Can you work these out from the model? Positions are in its coordinate system, mm. Give positions to 0.01 mm unless a question says otherwise; leave off trailing zeros. Loops run counter-clockwise (first coordinate to the right, second up) from the corner with the lowest first, then second, coordinate; pieces in that order, holes last. Notation, with made-up numbers: (85.25, -18.75) - (118.25, -18.75) arc R17 ccw to (118.25, 2.25) - close; hole circle Ø5 at (54.5, 33.25). An arc over 180 degrees is marked (long way). Answer as a JSON object with one key per item and string values. Group by question number.
Item 1: Suppose I cut it at A-A on x = -38.1. Write out the boundary of the cut face in (y, z), and give its area (3 significant figures).
Item 2: Thinking about a two-plate mould opening in X: for faces 1 (the cylindrical face through (0.58, -6.26, 60.23)), 2 (the flat face through (-12, 0, -7)), 3 (the cylindrical face through (2.753, -6.439, 56.765)), which applies, pulls with the +X half, pulls with the -X half, needs draft (parallel to the pull), parting line crosses it, or undercut?
Item 3: Suppose I cut it at D-D on z = -14. Write out the boundary of the cut face in (x, y).
Item 4: Suppose I cut it at B-B on x = 0. Write out the boundary of the cut face in (y, z), and give its area (3 significant figures).
Item 5: Will these pins go through, and if not, where does the flat tip stop? pin 1 (15 mm diameter, centred on x = 38.1, z = -21.62, fed in from -Y); pin 2 (4 mm diameter, centred on x = -28, y = -4, fed in from -Z); pin 3 (1 mm diameter, centred on y = -5, z = 4, fed in from -X); pin 4 (6 mm diameter, centred on x = -39.5, y = -11, fed in from +Z).
Item 6: Suppose I cut it at C-C on z = 11. Write out the boundary of the cut face in (x, y), and give its area (3 significant figures).
Item 7: Please list where these lines run through material, in increasing order: L1, parallel to Z at x = 0, y = -5.75; L2, parallel to Z at x = -38.1, y = -8.5; L3, parallel to X at y = -11, z = -22.
from build123d import *

# Parameters (mm, degrees)
F0_R     = 15.7260613119
F1_DEPTH = 12.7
F2_D     = 25.4


with BuildPart() as f1:
    # F0 (on Front) → F1 (new body)
    with BuildSketch(Plane.XZ):
        with BuildLine():
            ThreePointArc((-22.225, -21.624488881), (-24.3518467149, -13.686988881), (-30.1625, -7.8763355959))
            ThreePointArc((-30.1625, -7.8763355959), (-51.8481532851, -29.561988881), (-22.225, -21.624488881))
        make_face()
        with BuildLine():
            ThreePointArc((7.9375, 30.6184936023), (0, 28.4916468874), (-7.9375, 30.6184936023))
            ThreePointArc((-7.9375, 30.6184936023), (-15.8714708467, 9.5359543409), (-30.1625, -7.8763355959))
            ThreePointArc((-30.1625, -7.8763355959), (-24.3518467149, -13.686988881), (-22.225, -21.624488881))
            ThreePointArc((-22.225, -21.624488881), (0, -17.2054544996), (22.225, -21.624488881))
            ThreePointArc((22.225, -21.624488881), (24.3518467149, -13.686988881), (30.1625, -7.8763355959))
            ThreePointArc((30.1625, -7.8763355959), (15.3716015359, 9.2473546597), (7.9375, 30.6184936023))
        make_face()
        with Locations((0, 0.3947862569)):
            Circle(F0_R, mode=Mode.SUBTRACT)
        with BuildLine():
            ThreePointArc((53.975, -21.624488881), (46.0375, -7.8763355959), (30.1625, -7.8763355959))
            ThreePointArc((30.1625, -7.8763355959), (24.3518467149, -13.686988881), (22.225, -21.624488881))
            ThreePointArc((22.225, -21.624488881), (38.1, -37.499488881), (53.975, -21.624488881))
        make_face()
        with Locations((0, 0.3947862569)):
            Circle(F0_R)
        with BuildLine():
            ThreePointArc((7.9375, 30.6184936023), (13.7481532851, 36.4291468874), (15.875, 44.3666468874))
            ThreePointArc((15.875, 44.3666468874), (-7.9375, 58.1148001724), (-7.9375, 30.6184936023))
            ThreePointArc((-7.9375, 30.6184936023), (0, 28.4916468874), (7.9375, 30.6184936023))
        make_face()
    extrude(amount=F1_DEPTH)

    # F2 (through all)
    with Locations(Plane(origin=(0, 0, 0), x_dir=(1, 0, 0), z_dir=(0, 1, 0))):
        with Locations((-38.1, 21.624488881), (38.1, 21.624488881), (0, -44.3666468874), (0, -0.3947862569)):
            Hole(F2_D / 2)


solid = f1.part
Worked out:
{
 "1": {"outline": "(-12.7, -37.5) - (0, -37.5) - (0, -34.32) - (-12.7, -34.32) - close; (-12.7, -8.92) - (0, -8.92) - (0, -5.75) - (-12.7, -5.75) - close", "area": "80.6 mm2"},
 "2": {"face 1": "parting line crosses it", "face 2": "needs draft", "face 3": "undercut"},
 "3": {"outline": "(-52.02, -12.7) - (-48.26, -12.7) - (-48.26, 0) - (-52.02, 0) - close; (-27.94, -12.7) - (27.94, -12.7) - (27.94, 0) - (-27.94, 0) - close; (48.26, -12.7) - (52.02, -12.7) - (52.02, 0) - (48.26, 0) - close"},
 "4": {"outline": "(-12.7, -17.21) - (0, -17.21) - (0, -12.31) - (-12.7, -12.31) - close; (-12.7, 13.09) - (0, 13.09) - (0, 31.67) - (-12.7, 31.67) - close; (-12.7, 57.07) - (0, 57.07) - (0, 60.24) - (-12.7, 60.24) - close", "area": "338 mm2"},
 "5": {"pin 1": "passes through", "pin 2": "stops at z = -35.28", "pin 3": "stops at x = -19.79", "pin 4": "stops at z = -5.75"},
 "6": {"outline": "(-15.05, -12.7) - (-6.99, -12.7) - (-6.99, 0) - (-15.05, 0) - close; (6.99, -12.7) - (14.4, -12.7) - (14.4, 0) - (6.99, 0) - close", "area": "197 mm2"},
 "7": {"L1": "z = -17.21 to -12.31, 13.09 to 31.67, 57.07 to 60.24", "L2": "z = -37.5 to -34.32, -8.92 to -5.75", "L3": "x = -53.97 to -50.79, -25.41 to -22.23, 22.23 to 25.41, 50.79 to 53.97"}
}
